Can you work these out from the model? Positions are in its coordinate system, mm. Face numbers are marked on the shaded views. A direction names the side the tool comes from. Give positions to 0.01 mm unless a question says otherwise; leave off trailing zeros. Order: outer loops, then holes, each group sorted by start corner. A loop starts at its lowest first (then second) coordinate and runs counter-clockwise, first axis right, second up. Notation, with made-up numbers: (29.25, 57) - (44.25, 57) arc R26 ccw to (44.25, 88) - close; hole circle Ø7 at (70.5, 40). An arc over 180 degrees is marked (long way). Use one line per item in the form item = value. Start each with the question number.
1) Suppose I cut it at A-A, the plane z = 0. Write out the boundary of the cut face in (x, y) (3 decimals), and give its area (3 significant figures).
2) For pin 1 (2 mm diameter, centred on y = 9.5, z = 1.5, fed in from -X); pin 2 (4 mm diameter, centred on x = -4.5, z = -1.5, fed in from +Y), each with a flat end and sliding along its axis, tell me the tip position at first contact or that it passes through.
3) Suppose I cut it at D-D, the plane y = 9. Write out the boundary of the cut face in (x, z) (3 decimals), and give its area (3 significant figures).
4) Which directions (+Z, -Z, +X, -X, +Y, -Y) give clear straight access to the entire face, cutting with the end or side of a thin tool? Please do the marked faces 4, 5 and 6.
5) We'd pull the mould along Z, two halves only. Please class the marked faces 1, 2 and 3: released by +Z, released by -Z, zero draft, split by the parting line, or undercut.
6) Please list where these lines run through material, in increasing order: probe 1 along Y at (x, z) = (5.95, 0) (3 decimals); probe 2 along X at (y, z) = (1.9, 0) (3 decimals); probe 3 along Y at (x, z) = (3.25, 4).
7) Suppose I cut it at B-B, the plane x = 0. Write out the boundary of the cut face in (y, z) (3 decimals).
8) Suppose I cut it at C-C, the plane x = 7.5. Write out the boundary of the cut face in (y, z) (3 decimals), and give its area (3 significant figures).
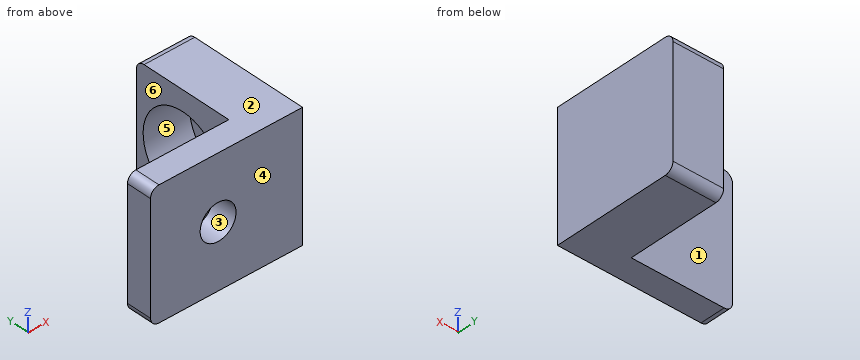
```python
from build123d import *

# Parameters (mm, degrees)
SKETCH_1_W          = 18
SKETCH_1_H          = 15
EXTRUDE_1_DEPTH     = 15
SKETCH_2_W          = 12
SKETCH_2_H          = 15
CUT_EXTRUDE_1_DEPTH = 12
FILLET_1_R          = 1
SKETCH_3_R          = 5.125
CUT_EXTRUDE_2_DEPTH = 5.5
SKETCH_4_R          = 2.125
CUT_EXTRUDE_3_DEPTH = 5.5


with BuildPart() as part:
    # 草圖1 → 填料-伸長1 (new body)
    with BuildSketch(Plane(origin=(0, 0, 0), x_dir=(1, 0, 0), z_dir=(0, 1, 0))):
        with Locations((1, 0)):
            Rectangle(SKETCH_1_W, SKETCH_1_H)
    extrude(amount=EXTRUDE_1_DEPTH)

    # 草圖2 → 除料-伸長1 (cut)
    with BuildSketch(Plane(origin=(0, 15, 0), x_dir=(1, 0, 0), z_dir=(0, 1, 0))):
        with Locations((-2, 0)):
            Rectangle(SKETCH_2_W, SKETCH_2_H)
    extrude(amount=-CUT_EXTRUDE_1_DEPTH, mode=Mode.SUBTRACT)

    # 圓角1
    fillet_1_edges = [part.edges().sort_by_distance(p)[0] for p in [
        (7, 15, 7.5),
        (-8, 1.5, -7.5),
        (-8, 1.5, 7.5),
        (7, 15, -7.5),
    ]]
    fillet(fillet_1_edges, radius=FILLET_1_R)

    # 草圖3 → 除料-伸長2 (cut)
    with BuildSketch(Plane.ZY.offset(-4)):
        with Locations((0, 9)):
            Circle(SKETCH_3_R)
    extrude(amount=-CUT_EXTRUDE_2_DEPTH, mode=Mode.SUBTRACT)

    # 草圖4 → 除料-伸長3 (cut)
    with BuildSketch(Plane(origin=(0, 3, 0), x_dir=(1, 0, 0), z_dir=(0, 1, 0))):
        with Locations(Location((0, 0, 0), (0, 0, 270))):
            Circle(SKETCH_4_R)
    extrude(amount=-CUT_EXTRUDE_3_DEPTH, mode=Mode.SUBTRACT)


solid = part.part
```
Result sheet:
q1.outline = (-8, 0) - (-2.125, 0) - (-2.125, 3) - (-8, 3) - close; (2.125, 0) - (10, 0) - (10, 15) - (4, 15) - (4, 14.125) - (9.5, 14.125) - (9.5, 3.875) - (4, 3.875) - (4, 3) - (2.125, 3) - close
q1.area = 56.9 mm²
q2.pin_1 = 9.5
q2.pin_2 = 3
q3.outline = (4, -7.5) - (10, -7.5) - (10, 7.5) - (4, 7.5) - (4, 5.125) - (9.5, 5.125) - (9.5, -5.125) - (4, -5.125) - close
q3.area = 33.6 mm²
q4.face_4 = +Z, -Z, +X, -X, -Y
q4.face_5 = -X
q4.face_6 = +Z, -Z, -X, +Y
q5.face_1 = zero draft
q5.face_2 = released by +Z
q5.face_3 = undercut
q6.probe_1 = 0 to 3.875, 14.125 to 15
q6.probe_2 = -8 to -2.125, 2.125 to 10
q6.probe_3 = 0 to 3
q7.outline = (0, -7.5) - (3, -7.5) - (3, -2.125) - (0, -2.125) - close; (0, 2.125) - (3, 2.125) - (3, 7.5) - (0, 7.5) - close
q8.outline = (0, -7.5) - (14, -7.5) arc R1 ccw to (15, -6.5) - (15, 6.5) arc R1 ccw to (14, 7.5) - (0, 7.5) - close; hole circle Ø10.25 at (9, 0)
q8.area = 142 mm²
